Could you check a few things on this drawing? It's one solid part, dimensions in mm from its lowest x, y, z. A direction names the side the tool comes from. Coordinates: 2 decimals unless noted, no trailing zeros. Loops run counter-clockwise (first coordinate to the right, second up) from the corner with the lowest first, then second, coordinate; pieces in that order, holes last. Notation, with made-up numbers: M -13.75,26.25 L 3.25,26.25 A11 cw 3.25,32.25 Z; hole C 0.25,30.25 d8. An arc over 180 degrees is marked long. Use one line per item in the form item = value. Start each with the question number.
(1) Imagine slicing it at D-D, the plane y = 2.75. Please give me the cut outline in (x, z), and give its area (3 significant figures).
(2) Imagine slicing it at B-B, the plane y = 16.75. Please give me the cut outline in (x, z), and give its area (3 significant figures).
(3) Thinking about a two-plate mould opening in Z: for the marked faces 1, 2, 3 and 4, which applies, +Z half, -Z half, draft (parallel to the pull), parting line (faces both ways), or undercut?
(4) Will these pins go through, and if not, where does the flat tip stop? P1, Ø2, axis at x = 3, z = 9, coming from the +Y side; P2, Ø2, axis at x = 11.5, z = 12, coming from the -Y side; P3, Ø1.5, axis at x = 7.5, z = 4.5, coming from the -Y side; P4, Ø1.5, axis at y = 16, z = 4, coming from the -X side (1 decimal).
(5) Please list where these lines run through material, in increasing order: L1, parallel to Y at x = 11, z = 2.75; L2, parallel to Y at x = 9, z = 6.5; L3, parallel to Z at x = 5.5, y = 1.25.
(6) On a 3-axis mill with a long thin cutter (end or side, diameter ignored), from which of +Z, -Z, +X, -X, +Y, -Y can I reach the whole of each face in a straight line? I mean the marked faces 5, 6 and 7. Say none if no direction works.
(7) Imagine slicing it at A-A, the plane z = 7. Please give me the cut outline in (x, y).
(8) Imagine slicing it at C-C, the plane x = 1.25. Please give me the cut outline in (y, z), and give its area (3 significant figures).
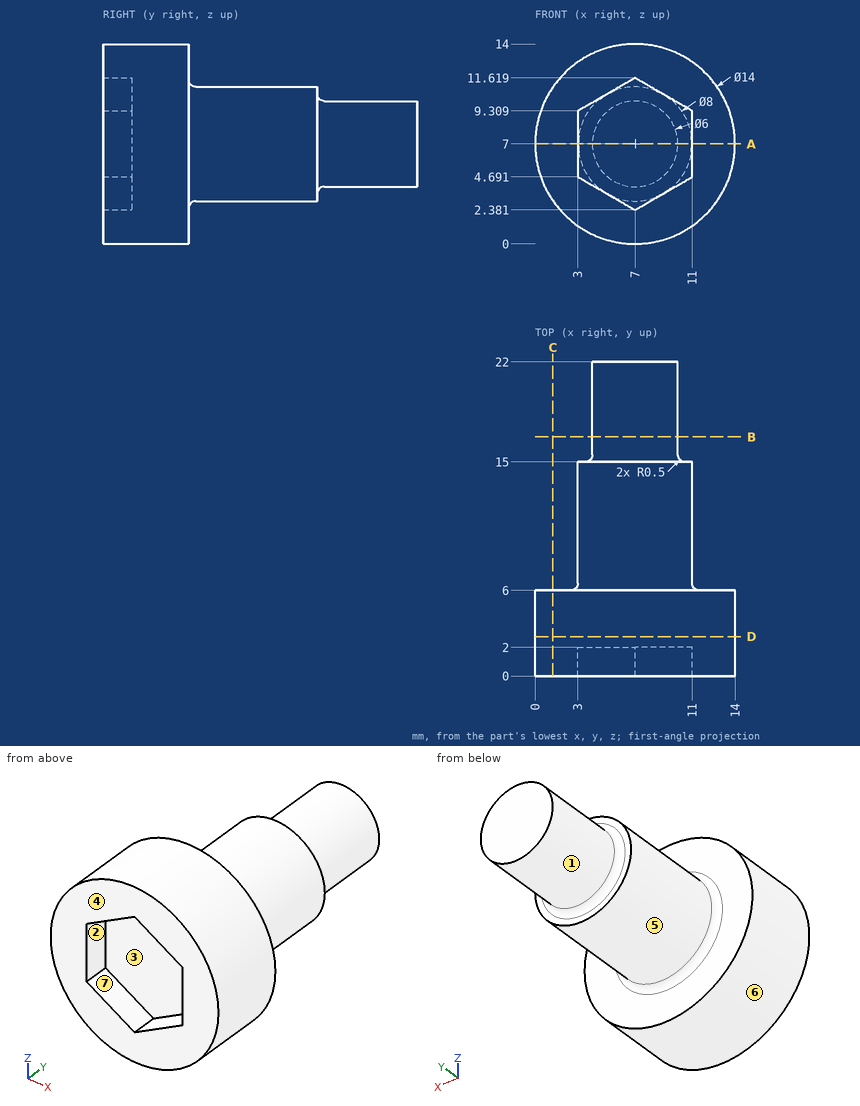
Answer:
q1.outline = C 7,7 d14
q1.area = 154 mm²
q2.outline = C 7,7 d6
q2.area = 28.3 mm²
q3.face_1 = parting line
q3.face_2 = undercut
q3.face_3 = undercut
q3.face_4 = draft
q4.P1 = 15
q4.P2 = 0
q4.P3 = 2
q4.P4 = 5
q5.L1 = 0 to 6
q5.L2 = 2 to 22
q5.L3 = 0.16 to 3.25, 10.75 to 13.84
q6.face_5 = +Y
q6.face_6 = +Y, -Y
q6.face_7 = -Y
q7.outline = M 0,0 L 3,0 L 3,2 L 11,2 L 11,0 L 14,0 L 14,6 L 11.5,6 A0.5 cw 11,6.5 L 11,15 L 10.5,15 A0.5 cw 10,15.5 L 10,22 L 4,22 L 4,15.5 A0.5 cw 3.5,15 L 3,15 L 3,6.5 A0.5 cw 2.5,6 L 0,6 Z
q8.outline = M 0,3.01 L 6,3.01 L 6,10.99 L 0,10.99 Z
q8.area = 47.9 mm²
